The model under review builds one solid part; all positions refer to its coordinate system, in mm. Give positions to 0.01 mm unless a question says otherwise; leave off trailing zeros. Loops run counter-clockwise (first coordinate to the right, second up) from the corner with the lowest first, then second, coordinate; pieces in that order, holes last. Notation, with made-up numbers: M -10.75,78.25 L -4.75,78.25 A19 cw -4.75,103.25 Z; hole C 16,64.5 d3. An arc over 180 degrees is marked long. Return JSON: item names as keys, results as strings.
```python
from build123d import *

# Parameters (mm, degrees)
SKETCH1_W             = 19.05
SKETCH1_H             = 29.5
BODY_DEPTH            = 31.75
SKETCH8_R             = 3.96875
AXLE_HOLE_DEPTH       = 40.856335757
F_6_32_TAPPED_HOLE1_D = 2.7051
ROUND_OVER_DEPTH      = 40.856335757
FILLET1_R             = 1.27


with BuildPart() as part:
    # Sketch1 → Body (new body)
    with BuildSketch(Plane(origin=(0, 0, 0), x_dir=(1, 0, 0), z_dir=(0, 1, 0))):
        Rectangle(SKETCH1_W, SKETCH1_H)
    extrude(amount=-BODY_DEPTH)

    # Sketch8 → Axle Hole (cut, through all)
    with BuildSketch(Plane.ZY.offset(9.525)):
        with Locations((0, -9.525)):
            Circle(SKETCH8_R)
    extrude(amount=-AXLE_HOLE_DEPTH, mode=Mode.SUBTRACT)

    # #6-32 Tapped Hole1 (through all)
    with Locations(Plane(origin=(0, -27.75, 14.75), x_dir=(1, 0, 0), z_dir=(0, 0, 1))):
        with Locations((0, 0), (0, 11.1125)):
            Hole(F_6_32_TAPPED_HOLE1_D / 2)

    # Sketch10 → Round Over (cut, through all)
    with BuildSketch(Plane(origin=(9.525, 0, 0), x_dir=(0, 0, -1), z_dir=(1, 0, 0))):
        with BuildLine():
            Line((-14.75, 0), (-14.75, -11.75))
            Line((-14.75, -11.75), (-9.261479363, -11.75))
            ThreePointArc((-9.261479363, -11.75), (-7.480599909, -3.628708793), (0, 0))
            Line((0, 0), (-14.75, 0))
        make_face()
        with BuildLine():
            Line((14.75, 0), (0, 0))
            ThreePointArc((0, 0), (6.735192091, -2.789807909), (9.525, -9.525))
            ThreePointArc((9.525, -9.525), (9.45889042, -10.645275427), (9.261479363, -11.75))
            Line((9.261479363, -11.75), (14.75, -11.75))
            Line((14.75, -11.75), (14.75, 0))
        make_face()
    extrude(amount=-ROUND_OVER_DEPTH, mode=Mode.SUBTRACT)

    # Fillet1
    fillet1_edges = [part.edges().sort_by_distance(p)[0] for p in [
        (-9.525, -31.75, 0),
        (0, -31.75, 14.75),
        (-9.525, -11.75, 12.005739682),
        (0, -11.75, 14.75),
        (9.525, -11.75, 12.005739682),
        (9.525, -31.75, 0),
        (-9.525, -11.75, -12.005739682),
        (0, -11.75, -14.75),
        (9.525, -11.75, -12.005739682),
        (0, -31.75, -14.75),
    ]]
    fillet(fillet1_edges, radius=FILLET1_R)


solid = part.part
```
1) Consider section A-A on z = 2. Count the separate pieces of the cut face and the enclosed holes in it, then the cut area to 3 significant figures.
From the geometry:
{"separate pieces": "2", "enclosed holes": "2", "area": "458 mm²"}
2) Wall thickness on L1, parallel to Y at x = 0, z = 5; L2, parallel to Y at x = 0, z = -3.25; L3, parallel to Y at x = 0, z = 6.5: over which ranges is each line inside the solid? List them lowest first. Write a range as from..to.
From the geometry:
{"L1": "-31.75..-29.1, -26.4..-17.99, -15.28..-1.42", "L2": "-31.75..-29.1, -26.4..-17.99, -15.28..-11.8, -7.25..-0.57", "L3": "-31.75..-29.1, -26.4..-17.99, -15.28..-2.56"}
3) Consider section B-B on y = -27.75. Write out the cut boundary in (x, z) (3 decimals), then the cut area to 3 significant figures.
From the geometry:
{"outline": "M -9.525,-14.75 L -1.353,-14.75 L -1.353,14.75 L -9.525,14.75 Z; M 1.353,-14.75 L 9.525,-14.75 L 9.525,14.75 L 1.353,14.75 Z", "area": "482 mm²"}
4) Insertion check: pin 1 (4.5 mm diameter, centred on x = -3.5, z = -11, fed in from +Y); pin 2 (8 mm diameter, centred on x = 7, z = 4, fed in from +Y). Each pin has a flat end and moves straight along its axis. Give the tip position at first contact, or say it passes through.
From the geometry:
{"pin 1": "y = -5.76", "pin 2": "y = 0"}
5) The part is to be moulded in two halves that separate along X. For faces 1 (the face through (-0.62, -28.95, -0.21)), 2 (the face through (-9.16, -31.37, -0.21)), 3 (the face through (9.525, -18, 0)), say which applies: released by +X, released by -X, zero draft, split by the parting line, or undercut.
From the geometry:
{"face 1": "undercut", "face 2": "released by -X", "face 3": "released by +X"}
